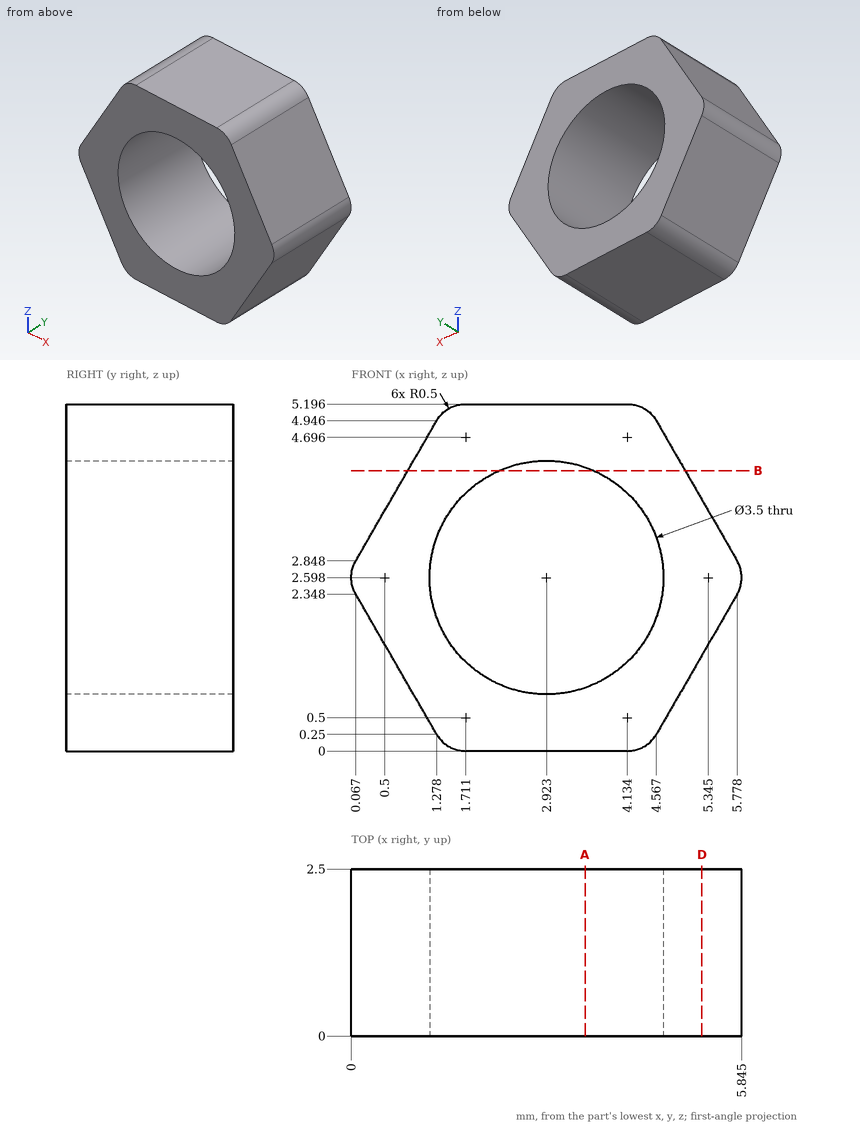
For this review, use the dimensioned drawing (mm, ordinates from the lowest corner) and the shaded views. Coordinates: 2 decimals unless noted, no trailing zeros. Loops run counter-clockwise (first coordinate to the right, second up) from the corner with the lowest first, then second, coordinate; pieces in that order, holes last. Notation, with made-up numbers: (79, -29) -> (136, -29) arc R36 cw to (136, 9) -> close; hole circle Ø4 at (-32.5, 36.5). An arc over 180 degrees is marked (long way). Use a Markdown table: item, result. Add a question column.
1. Add section B-B on z = 4.2. Write out the cut boundary in (x, y).
2. Add section A-A on x = 3.5. Write out the cut boundary in (y, z).
3. Clearance check with flat-ended pins moving along their axes: pin 1 Ø1 at (y, z) = (1, 2) entering from +X (1 decimal); pin 2 Ø1.5 at (y, z) = (1, 1.5) entering from -X. State where each tip first meets the part, or that it passes through.
4. To check wall thickness, follow line 1 (Z direction, x = 2.9, y = 0.95); line 2 (Z direction, x = 2.3, y = 0.2) (1 decimal); line 3 (X direction, y = 0.9, z = 3.1) (1 decimal). State the ranges of each line that lie inside material, in increasing order.
5. Add section D-D on x = 5.25. Write out the cut boundary in (y, z).
Returned:
| question | item | result |
|---|---|---|
| 1 | outline | (0.85, 0) -> (2.22, 0) -> (2.22, 2.5) -> (0.85, 2.5) -> close; (3.63, 0) -> (5, 0) -> (5, 2.5) -> (3.63, 2.5) -> close |
| 2 | outline | (0, 0) -> (2.5, 0) -> (2.5, 0.95) -> (0, 0.95) -> close; (0, 4.25) -> (2.5, 4.25) -> (2.5, 5.2) -> (0, 5.2) -> close |
| 3 | pin 1 | stops at x = 5.8 |
| 3 | pin 2 | stops at x = 0.12 |
| 4 | line 1 | z = 0 to 0.85, 4.35 to 5.2 |
| 4 | line 2 | z = 0 to 1, 4.2 to 5.2 |
| 4 | line 3 | x = 0.2 to 1.2, 4.6 to 5.6 |
| 5 | outline | (0, 1.43) -> (2.5, 1.43) -> (2.5, 3.76) -> (0, 3.76) -> close |
